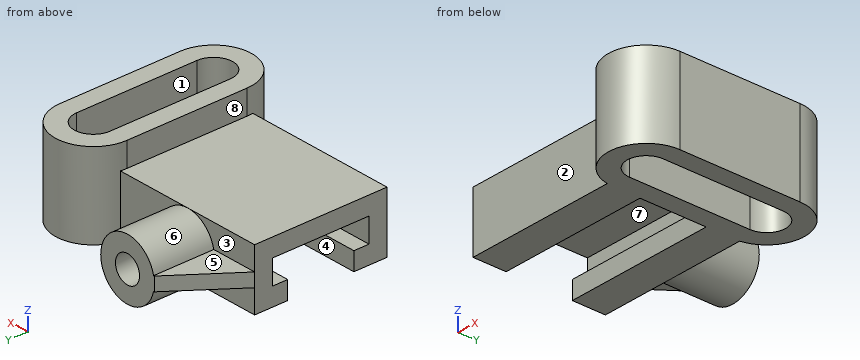
from build123d import *

# Parameters (mm, degrees)
BOSS_EXTRUDE1_DEPTH        = 56
BOSS_EXTRUDE2_START        = -0.322075
BOSS_EXTRUDE2_DEPTH        = 100.322075
SKETCH5_R                  = 20
BOSS_EXTRUDE3_DEPTH        = 40
RIB7_START                 = -4.5
RIB7_DEPTH                 = 9
F_12_0MM_DOWEL_HOLE1_D     = 18
F_12_0MM_DOWEL_HOLE1_DEPTH = 32


with BuildPart() as part:
    # Sketch3 → Boss-Extrude1 (new body)
    with BuildSketch(Plane.XY):
        with BuildLine():
            Line((25, 40), (25, -40))
            ThreePointArc((25, -40), (0, -65), (-25, -40))
            Line((-25, -40), (-25, 40))
            ThreePointArc((-25, 40), (0, 65), (25, 40))
        make_face()
        with BuildLine():
            Line((12.5, 40), (12.5, -40))
            ThreePointArc((12.5, -40), (0, -52.5), (-12.5, -40))
            Line((-12.5, -40), (-12.5, 40))
            ThreePointArc((-12.5, 40), (0, 52.5), (12.5, 40))
        make_face(mode=Mode.SUBTRACT)
    extrude(amount=BOSS_EXTRUDE1_DEPTH)

    # Sketch4 → Boss-Extrude2 (add)
    with BuildSketch(Plane.ZY.offset(25).offset(BOSS_EXTRUDE2_START)):
        Polygon((12, 22), (0, 22), (0, 44), (40, 44), (40, -44), (0, -44), (0, -22), (12, -22), (12, -32), (28, -32), (28, 32), (12, 32), align=None)
    extrude(amount=BOSS_EXTRUDE2_DEPTH)

    # Sketch5 → Boss-Extrude3 (add)
    with BuildSketch(Plane(origin=(0, 44, 0), x_dir=(1, 0, 0), z_dir=(0, 1, 0))):
        with Locations(Location((-75, -20, 0), (0, 0, 270))):
            Circle(SKETCH5_R)
    extrude(amount=BOSS_EXTRUDE3_DEPTH)

    # Rib7: read off the stored shape, not the designer's step
    # Rib7 outline → Rib7 (add)
    with BuildSketch(Plane.XY.offset(20).offset(RIB7_START)):
        Polygon((-125, 44), (-94.48717527, 44), (-94.48717527, 84), (-95, 84), align=None)
    extrude(amount=RIB7_DEPTH)

    # Ø12.0mm Dowel Hole1
    with Locations(Plane(origin=(-75, 84, 20), x_dir=(0, 0, 1), z_dir=(0, 1, 0))):
        with Locations((0, 0)):
            Hole(F_12_0MM_DOWEL_HOLE1_D / 2, depth=F_12_0MM_DOWEL_HOLE1_DEPTH)


solid = part.part
Source: CAD feature listing. Evaluate the final solid. Frame: model axes, mm. Face numbers are marked on the shaded views. A direction names the side the tool comes from. Round coordinates to 2 decimals unless told otherwise and drop trailing zeros. Loops run counter-clockwise (first coordinate to the right, second up) from the corner with the lowest first, then second, coordinate; pieces in that order, holes last. Notation, with made-up numbers: M 32,-24.75 L 76,-24.75 A18 cw 76,-13.75 Z; hole C 26.25,63.5 d3. An arc over 180 degrees is marked long. Return JSON: item names as keys, results as strings. Group by question number.
1. Section query B-B on z = 20. Output: boundary loops of the cut face in (x, y).
2. Section query A-A on y = -30. Output: boundary loops of the cut face in (x, z), and give its area (3 significant figures).
3. Mould query, pull axis Y, two halves, no side actions, for the marked faces 1, 2, 3 and 4. Classes: released by +Y, released by -Y, zero draft, split by the parting line, or undercut.
4. Reachability of the marked faces 5, 6, 7 and 8 from +Z, -Z, +X, -X, +Y, -Y: full face, straight path, thin tool, end or side. Return the list, or none.
5. Material intervals for line 1 along X through (y, z) = (15.5, 17); line 2 along Y through (x, z) = (-85.5, 7); line 3 along Y through (x, z) = (-0.5, 30) (3 decimals), sorted ascending. Write a range as from..to.
6. Section query D-D on y = 34.5. Output: boundary loops of the cut face in (x, z), and give its area (3 significant figures).
7. Section query C-C on x = -10. Output: boundary loops of the cut face in (y, z).
8. Pin query (flat end, axial travel): pin 1 (11 mm diameter, centred on x = -75, z = 20, fed in from -Y); pin 2 (8 mm diameter, centred on x = -16.5, z = 33, fed in from -Y); pin 3 (6 mm diameter, centred on x = -26, z = 35.5, fed in from +Y). Return the tip coordinate at first contact, or that it passes through.
Checks:
{
 "1": {"outline": "M -125,-44 L -24.68,-44 A25 ccw 25,-40 L 25,40 A25 ccw -24.68,44 L -55,44 L -55,84 L -66,84 L -66,52 L -84,52 L -84,84 L -95,84 L -125,44 L -125,32 L -25,32 L -25,-32 L -125,-32 Z; hole M -12.5,-40 A12.5 ccw 12.5,-40 L 12.5,40 A12.5 ccw -12.5,40 Z"},
 "2": {"outline": "M -125,0 L -12.5,0 L -12.5,56 L -25,56 L -25,40 L -125,40 L -125,28 L -25,28 L -25,12 L -125,12 Z; M 12.5,0 L 25,0 L 25,56 L 12.5,56 Z", "area": "3,800 mm²"},
 "3": {"face 1": "undercut", "face 2": "released by -Y", "face 3": "released by +Y", "face 4": "undercut"},
 "4": {"face 5": "+Z, -X, +Y", "face 6": "+Y", "face 7": "-X", "face 8": "+Z, -X, +Y, -Y"},
 "5": {"line 1": "x = -25..-12.5, 12.5..25", "line 2": "y = -44..-22, 22..84", "line 3": "y = -64.995..-52.49, 52.49..64.995"},
 "6": {"outline": "M -125,0 L -12.5,0 L -12.5,56 L -25,56 L -25,40 L -125,40 Z; M 12.5,0 L 25,0 L 25,56 L 12.5,56 Z", "area": "5,400 mm²"},
 "7": {"outline": "M -62.91,0 L -47.5,0 L -47.5,56 L -62.91,56 Z; M 47.5,0 L 62.91,0 L 62.91,56 L 47.5,56 Z"},
 "8": {"pin 1": "stops at y = -44", "pin 2": "stops at y = -61.65", "pin 3": "stops at y = 49.8"}
}
